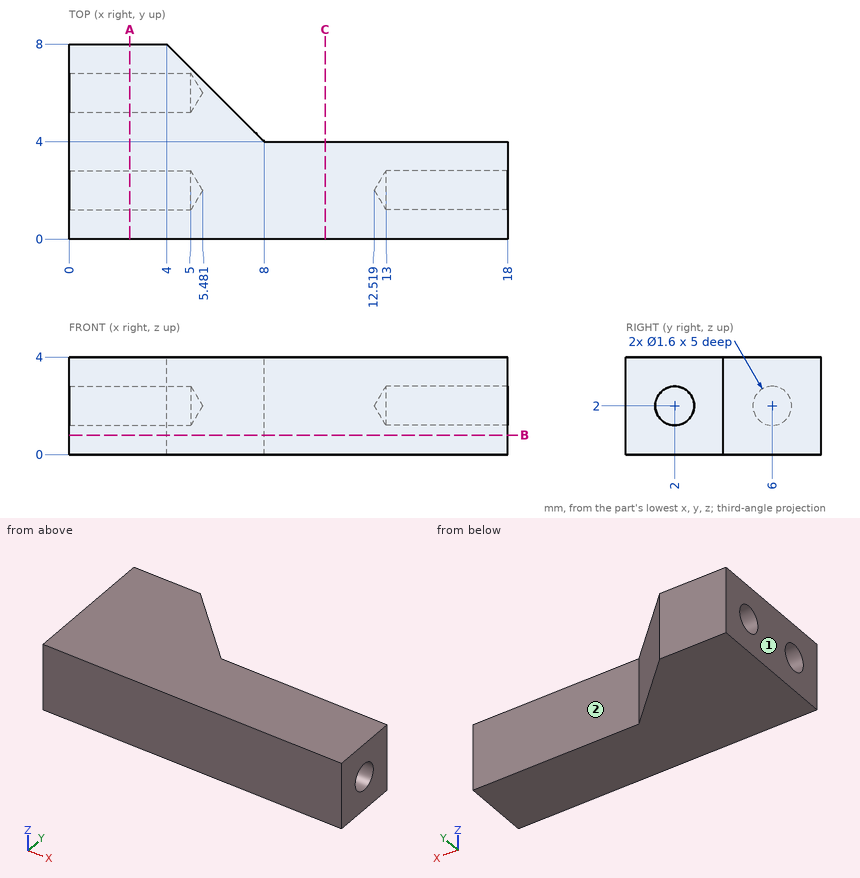
Answer from the drawing. Dimensions are ordinates in mm from the lowest x, y and z of the part. A direction names the side the tool comes from. Coordinates: 2 decimals unless noted, no trailing zeros. Write each loop counter-clockwise with the first axis right and the second up, starting at its lowest first coordinate (ties: lowest second). Pieces come first, ordered by that corner, then holes. Notation, with made-up numbers: (29, 28.5) - (69, 28.5) arc R23 ccw to (69, 63.5) - close; hole circle Ø11 at (1.5, -36.5). An arc over 180 degrees is marked (long way). Return JSON: item names as keys, results as strings. Group by question number.
Q1. Flat-ended cylindrical pins translate along their axes: pin 1 Ø1 at (y, z) = (6, 2) entering from +X; pin 2 Ø2 at (x, z) = (15.5, 1.5) entering from +Y. Find the tip coordinate at first contact, or state that the pin passes through.
Q2. The part is cut by section A-A on x = 2.5. Write down the section's boundary in (y, z).
Q3. Find the intervals of material crossed by line 1 along Y through (x, z) = (3.5, 2); line 2 along Z through (x, y) = (1.25, 6); line 3 along Y through (x, z) = (11.25, 1), in increasing order. Write a range as [from, to].
Q4. The part is cut by section C-C on x = 10.5. Write down the section's boundary in (y, z).
Q5. Which of the six approach directions +Z, -Z, +X, -X, +Y, -Y give full straight-line access (tool end or side, diameter ignored) to the marked faces 1 and 2?
Q6. The part is cut by section B-B on z = 0.8. Write down the section's boundary in (x, y), and give its area (3 significant figures).
Evaluation:
{
 "1": {"pin 1": "stops at x = 6.5", "pin 2": "stops at y = 4"},
 "2": {"outline": "(0, 0) - (8, 0) - (8, 4) - (0, 4) - close; hole circle Ø1.6 at (2, 2); hole circle Ø1.6 at (6, 2)"},
 "3": {"line 1": "y = [0, 1.2], [2.8, 5.2], [6.8, 8]", "line 2": "z = [0, 1.2], [2.8, 4]", "line 3": "y = [0, 4]"},
 "4": {"outline": "(0, 0) - (4, 0) - (4, 4) - (0, 4) - close"},
 "5": {"face 1": "+Z, -Z, -X, +Y, -Y", "face 2": "+Z, -Z, +X, +Y"},
 "6": {"outline": "(0, 0) - (18, 0) - (18, 4) - (8, 4) - (4, 8) - (0, 8) - close", "area": "96.0 mm2"}
}
